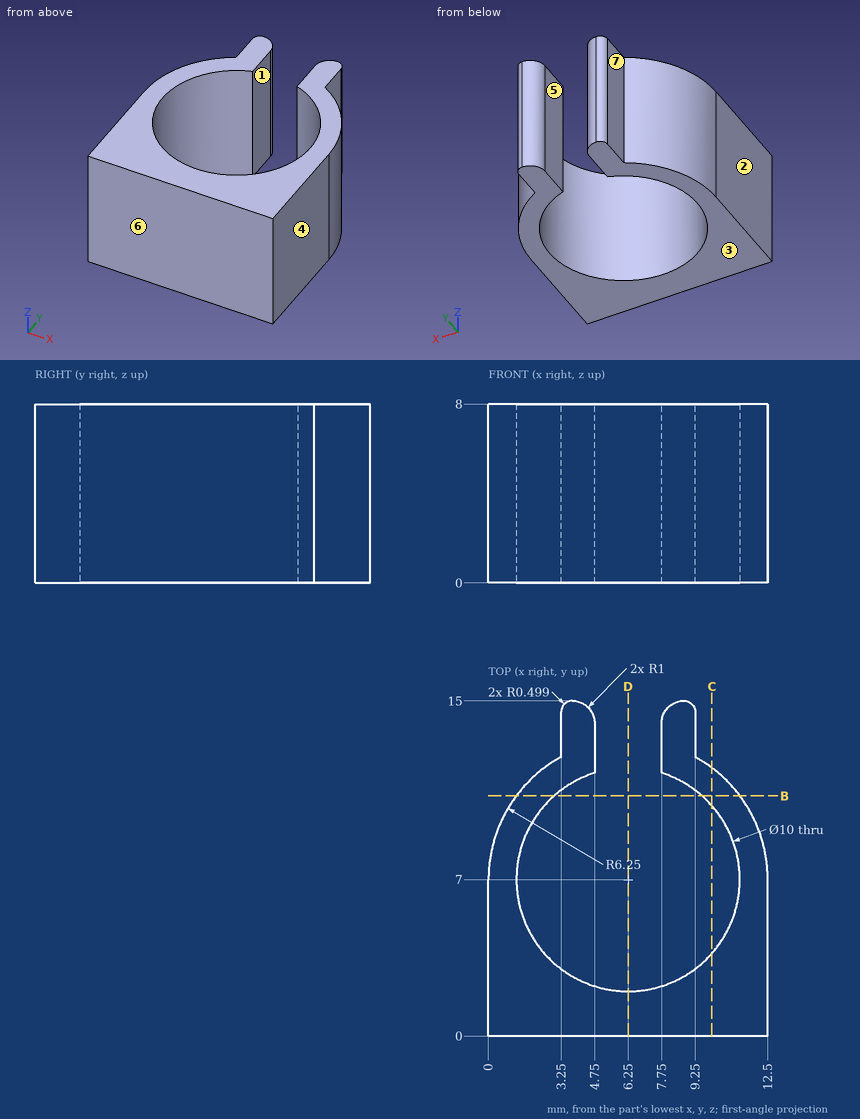
Design review of the part shown in the three views and the two pictorial views. Dimensions are in mm from the part's minimum x, y and z. A direction names the side the tool comes from. Round coordinates to 2 decimals unless told otherwise and drop trailing zeros. Loops run counter-clockwise (first coordinate to the right, second up) from the corner with the lowest first, then second, coordinate; pieces in that order, holes last.
1) Consider section D-D on x = 6.25. State the section outline as (y, z) points.
Values follow:
outline: (0, 0) - (2, 0) - (2, 8) - (0, 8) - close
2) Consider section B-B on y = 10.75. State the section outline as (x, z) points.
Values follow:
outline: (1.25, 0) - (2.94, 0) - (2.94, 8) - (1.25, 8) - close; (9.56, 0) - (11.25, 0) - (11.25, 8) - (9.56, 8) - close
3) Tool access review of the marked faces 5, 6 and 7: name each direction out of +Z, -Z, +X, -X, +Y, -Y from which nothing blocks a thin tool from reaching the whole face with its end or side.
Values follow:
face 5: +Z, -Z, +Y
face 6: +Z, -Z, +X, -X, -Y
face 7: +Z, -Z, -X, +Y
4) Wall thickness on line 1 along X through (y, z) = (7, 5.5); line 2 along X through (y, z) = (12.75, 4.25); line 3 along Y through (x, z) = (4.5, 2.5) (1 decimal): over which ranges is each line inside the solid? List them lowest first.
Values follow:
line 1: x = 0 to 1.25, 11.25 to 12.5
line 2: x = 3.25 to 4.75, 7.75 to 9.25
line 3: y = 0 to 2.3, 11.7 to 14.7
5) Consider section C-C on x = 10. State the section outline as (y, z) points.
Values follow:
outline: (0, 0) - (3.69, 0) - (3.69, 8) - (0, 8) - close; (10.31, 0) - (12, 0) - (12, 8) - (10.31, 8) - close
6) The part is to be moulded in two halves that separate along X. For the marked faces 1, 2, 3 and 4, say which applies: pulls with the +X half, pulls with the -X half, needs draft (parallel to the pull), parting line crosses it, or undercut.
Values follow:
face 1: undercut
face 2: pulls with the -X half
face 3: needs draft
face 4: pulls with the +X half
7) Clearance check with flat-ended pins moving along their axes: P1, Ø1, axis at x = 2.5, z = 3.5, coming from the -Y side; P2, Ø6, axis at x = 6.25, y = 7, coming from the +Z side; P3, Ø0.7, axis at y = 12.5, z = 4, coming from the -X side; P4, Ø1, axis at y = 13.5, z = 5.5, coming from the -X side. State where each tip first meets the part, or that it passes through.
Values follow:
P1: stops at y = 0
P2: passes through
P3: stops at x = 2.71
P4: stops at x = 3.25
